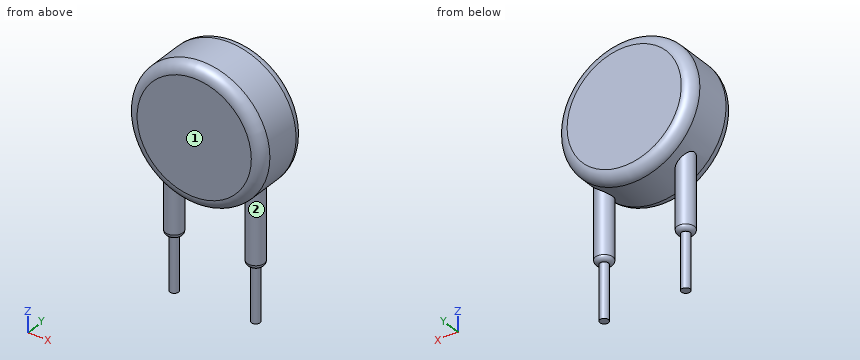
from build123d import *

# Parameters (mm, degrees)
F0_R     = 6.25
F1_DEPTH = 2.7
F2_R     = 0.8
F2_R_2   = 0.4
F4_DEPTH = 5
F5_R     = 0.39999
F6_R     = 1


# Not quite as in the source:
# - a fillet or chamfer is up to 0.001 mm smaller than in the source, because OpenCascade refuses the exact size
# - a feature names something its author has since deleted; it is built from what else it names


with BuildPart() as f1:
    # F0 (on Front) → F1 (new body, symmetric)
    with BuildSketch(Plane.XZ):
        with Locations((0, 11.25)):
            Circle(F0_R)
    extrude(amount=F1_DEPTH, both=True)

    # F2 (on Top) → F3 (join, up to the next surface of F1)
    with BuildSketch(Plane.XY):
        with Locations((-3.75, 0)):
            Circle(F2_R)
        with Locations((-3.75, 0)):
            Circle(F2_R_2, mode=Mode.SUBTRACT)
        with Locations((3.75, 0)):
            Circle(F2_R)
        with Locations((3.75, 0)):
            Circle(F2_R_2, mode=Mode.SUBTRACT)
        with Locations((-3.75, 0)):
            Circle(F2_R_2)
        with Locations((3.75, 0)):
            Circle(F2_R_2)
    extrude(until=Until.NEXT)

    # F2 (on Top) → F4 (join)
    with BuildSketch(Plane.XY):
        with Locations((-3.75, 0)):
            Circle(F2_R_2)
        with Locations((3.75, 0)):
            Circle(F2_R_2)
    extrude(amount=-F4_DEPTH)

    # F5 (radius 0.4 in the source; OpenCascade refuses exactly that, so slightly less here)
    f5_edges = [f1.edges().sort_by_distance(p)[0] for p in [
        (-4.55, 0, 0),
        (2.95, 0, 0),
    ]]
    fillet(f5_edges, radius=F5_R)

    # F6
    f6_edges = [f1.edges().sort_by_distance(p)[0] for p in [
        (-6.25, -2.7, 11.25),
        (-6.25, 2.7, 11.25),
    ]]
    fillet(f6_edges, radius=F6_R)


solid = f1.part
Geometry: final body of the model. Coordinates: model frame, mm. Face numbers are marked on the shaded views. A direction names the side the tool comes from. Coordinates: 2 decimals unless noted, no trailing zeros. Write each loop counter-clockwise with the first axis right and the second up, starting at its lowest first coordinate (ties: lowest second). Pieces come first, ordered by that corner, then holes. Notation, with made-up numbers: (6, -37.5) - (28, -37.5) arc R13 cw to (28, -29.5) - close; hole circle Ø9 at (-21.75, 6.25). An arc over 180 degrees is marked (long way). Return JSON: item names as keys, results as strings.
Item 1: Line query: L1, parallel to X at y = 0.4, z = 0.75; L2, parallel to X at y = -0.3, z = 4; L3, parallel to Z at x = -0.25, y = -0.1 (3 decimals). Output: solid intervals per line, ascending.
Completed:
{"L1": "x = -4.44 to -3.06, 3.06 to 4.44", "L2": "x = -4.49 to -3.01, 3.01 to 4.49", "L3": "z = 5.005 to 17.495"}
Item 2: Pin query (flat end, axial travel): pin 1 Ø1.5 at (x, y) = (2, 0.5) entering from +Z; pin 2 Ø2 at (x, y) = (1.5, 1.5) entering from +Z; pin 3 Ø1.5 at (x, y) = (4.5, -0.5) entering from +Z. Return the tip coordinate at first contact, or that it passes through.
Completed:
{"pin 1": "stops at z = 17.37", "pin 2": "stops at z = 17.48", "pin 3": "stops at z = 16.25"}
Item 3: Section query A-A (x = 0). Output: boundary loops of the cut face in (y, z).
Completed:
{"outline": "(-2.7, 6) arc R1 ccw to (-1.7, 5) - (1.7, 5) arc R1 ccw to (2.7, 6) - (2.7, 16.5) arc R1 ccw to (1.7, 17.5) - (-1.7, 17.5) arc R1 ccw to (-2.7, 16.5) - close"}
Item 4: Section query C-C (z = 3). Output: boundary loops of the cut face in (x, y).
Completed:
{"outline": "circle Ø1.6 at (-3.75, 0); circle Ø1.6 at (3.75, 0)"}
Item 5: Reachability of the marked faces 1 and 2 from +Z, -Z, +X, -X, +Y, -Y: full face, straight path, thin tool, end or side. Return the list, or none.
Completed:
{"face 1": "+Z, -Z, +X, -X, -Y", "face 2": "-Z"}
